Geometry check sheet. Reference: the model listing, model coordinates, mm. Face numbers are marked on the shaded views. Round coordinates to 2 decimals unless told otherwise and drop trailing zeros. Write each loop counter-clockwise with the first axis right and the second up, starting at its lowest first coordinate (ties: lowest second). Pieces come first, ordered by that corner, then holes. Notation, with made-up numbers: M 12.5,66 L 69.5,66 A9 cw 69.5,76 Z; hole C -17.75,-37.5 d8. An arc over 180 degrees is marked long. One line per item, written item: value. Start each with the question number.
1. Section check C-C (x = 19.05). Record the boundary of the cut face in (y, z) (3 decimals), and give its area (3 significant figures).
2. Section check D-D (y = 5.25). Record the boundary of the cut face in (x, z) (3 decimals).
3. Section check A-A (y = 0). Record the boundary of the cut face in (x, z) (3 decimals), and give its area (3 significant figures).
4. Release check for a two-part mould opening along Y. For the marked faces 1, 2 and 3 record: pulls with the +Y half, pulls with the -Y half, needs draft (parallel to the pull), parting line crosses it, or undercut.
5. Scan lines: probe 1 along X at (y, z) = (0.25, 16.75); probe 2 along X at (y, z) = (6.75, 11.25); probe 3 along X at (y, z) = (-2.5, 8.75). Record each from-to range of solid material in increasing order. Write a range as [from, to].
6. Section check B-B (z = 11.75). Record the boundary of the cut face in (x, y) (3 decimals), and give its area (3 significant figures).
7. Depth check by flat-ended pin: P1, Ø4, axis at x = 0, z = 9.525, coming from the -Y side. Enter the tip coordinate at first touch or a pass-through.
from build123d import *

# Parameters (mm, degrees)
SKETCH1_W               = 76.2
SKETCH1_H               = 19.05
BOSS_EXTRUDE1_DEPTH     = 19.05
F_1_4_CLEARANCE_HOLE1_D = 6.7564
F_1_4_CLEARANCE_HOLE2_D = 6.7564


with BuildPart() as part:
    # Sketch1 → Boss-Extrude1 (new body)
    with BuildSketch(Plane.XY):
        Rectangle(SKETCH1_W, SKETCH1_H)
    extrude(amount=BOSS_EXTRUDE1_DEPTH)

    # 1/4 Clearance Hole1 (through all)
    with Locations(Plane.XY.offset(19.05)):
        with Locations((-28.575, 0), (28.575, 0)):
            Hole(F_1_4_CLEARANCE_HOLE1_D / 2)

    # 1/4 Clearance Hole2 (through all)
    with Locations(Plane(origin=(0, 9.525, 0), x_dir=(1, 0, 0), z_dir=(0, 1, 0))):
        with Locations((0, -9.525), (-19.05, -9.525), (19.05, -9.525)):
            Hole(F_1_4_CLEARANCE_HOLE2_D / 2)


solid = part.part
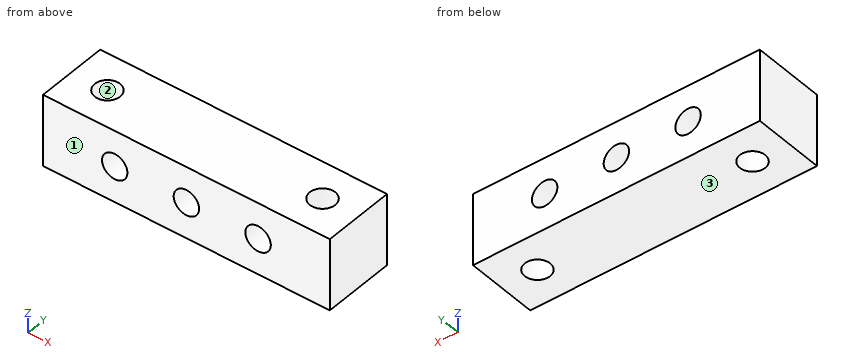
Result sheet:
1. outline: M -9.525,0 L 9.525,0 L 9.525,6.147 L -9.525,6.147 Z; M -9.525,12.903 L 9.525,12.903 L 9.525,19.05 L -9.525,19.05 Z
1. area: 234 mm2
2. outline: M -38.1,0 L 38.1,0 L 38.1,19.05 L -38.1,19.05 Z; hole C -19.05,9.525 d6.756; hole C 0,9.525 d6.756; hole C 19.05,9.525 d6.756
3. outline: M -38.1,0 L -31.953,0 L -31.953,19.05 L -38.1,19.05 Z; M -25.197,0 L 25.197,0 L 25.197,19.05 L -25.197,19.05 Z; M 31.953,0 L 38.1,0 L 38.1,19.05 L 31.953,19.05 Z; hole C -19.05,9.525 d6.756; hole C 0,9.525 d6.756; hole C 19.05,9.525 d6.756
3. area: 1,090 mm2
4. face 1: pulls with the -Y half
4. face 2: undercut
4. face 3: needs draft
5. probe 1: x = [-38.1, -31.94], [-25.21, 25.21], [31.94, 38.1]
5. probe 2: x = [-38.1, -21.95], [-16.15, -2.9], [2.9, 16.15], [21.95, 38.1]
5. probe 3: x = [-38.1, -30.85], [-26.3, -22.34], [-15.76, -3.29], [3.29, 15.76], [22.34, 26.3], [30.85, 38.1]
6. outline: M -38.1,-9.525 L -21.592,-9.525 L -21.592,9.525 L -38.1,9.525 Z; M -16.508,-9.525 L -2.542,-9.525 L -2.542,9.525 L -16.508,9.525 Z; M 2.542,-9.525 L 16.508,-9.525 L 16.508,9.525 L 2.542,9.525 Z; M 21.592,-9.525 L 38.1,-9.525 L 38.1,9.525 L 21.592,9.525 Z; hole C -28.575,0 d6.756; hole C 28.575,0 d6.756
6. area: 1,090 mm2
7. P1: passes through
